The model under review builds one solid part; all positions refer to its coordinate system, in mm. Coordinates: 2 decimals unless noted, no trailing zeros. Write each loop counter-clockwise with the first axis right and the second up, starting at its lowest first coordinate (ties: lowest second). Pieces come first, ordered by that corner, then holes. Notation, with made-up numbers: (-2, -17.75) - (43, -17.75) arc R7 cw to (43, -11.75) - close; hole circle Ø5 at (16, -24.5). An arc over 180 degrees is marked (long way). Put each result on its own line as item: value.
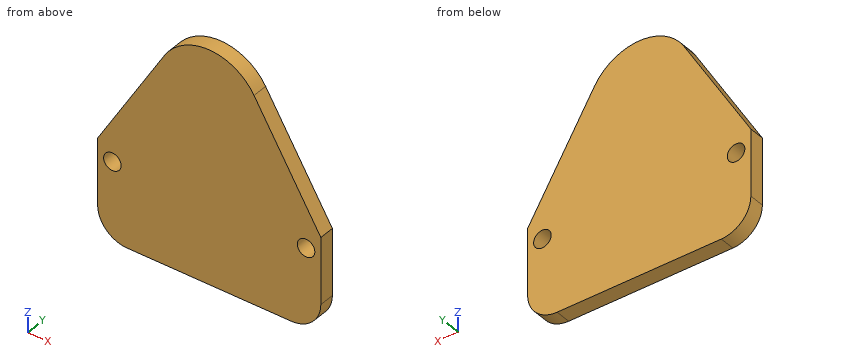
from build123d import *

# Parameters (mm, degrees)
SKETCH1_R           = 2.375
BOSS_EXTRUDE1_DEPTH = 4.15


with BuildPart() as part:
    # Sketch1 → Boss-Extrude1 (new body)
    with BuildSketch(Plane(origin=(0, 0, 0), x_dir=(1, 0, 0), z_dir=(0, 1, 0))):
        with BuildLine():
            Line((-22.25, 31.5), (22.25, 31.5))
            ThreePointArc((22.25, 31.5), (27.906854249, 29.156854249), (30.25, 23.5))
            Line((30.25, 23.5), (30.25, 5.5))
            Line((30.25, 5.5), (12.147813291, -24.627097925))
            ThreePointArc((12.147813291, -24.627097925), (0, -31.5), (-12.147813291, -24.627097925))
            Line((-12.147813291, -24.627097925), (-30.25, 5.5))
            Line((-30.25, 5.5), (-30.25, 23.5))
            ThreePointArc((-30.25, 23.5), (-27.906854249, 29.156854249), (-22.25, 31.5))
        make_face()
        with Locations(Location((26.25, 10.1, 0), (0, 0, 90))):
            Circle(SKETCH1_R, mode=Mode.SUBTRACT)
        with Locations(Location((-26.25, 10.1, 0), (0, 0, 90))):
            Circle(SKETCH1_R, mode=Mode.SUBTRACT)
    extrude(amount=BOSS_EXTRUDE1_DEPTH)


solid = part.part
1. Consider section C-C on x = 26.25. State the section outline as (y, z) points (3 decimals), plus the area to 3 significant figures.
Determined:
outline: (0, -30.428) - (4.15, -30.428) - (4.15, -12.475) - (0, -12.475) - close; (0, -7.725) - (4.15, -7.725) - (4.15, 1.157) - (0, 1.157) - close
area: 111 mm^2
2. For pin 1 Ø2 at (y, z) = (3, 24.5) entering from +X; pin 2 Ø4.5 at (x, z) = (26.25, -10.1) entering from +Y, all flat-tipped, find the tip position at first contact; note any pin that passes through.
Determined:
pin 1: stops at x = 12.83
pin 2: passes through
3. To check wall thickness, follow probe 1 along X at (y, z) = (1.15, -10.1) (3 decimals); probe 2 along Z at (x, y) = (24.5, 1.2); probe 3 along Z at (x, y) = (-26.25, 1.3) (3 decimals). State the ranges of each line that lie inside material, in increasing order.
Determined:
probe 1: x = -30.25 to -28.625, -23.875 to 23.875, 28.625 to 30.25
probe 2: z = -31.18 to -11.71, -8.49 to 4.07
probe 3: z = -30.428 to -12.475, -7.725 to 1.157
4. Consider section D-D on x = -25. State the section outline as (y, z) points, plus the area to 3 significant figures.
Determined:
outline: (0, -31.01) - (4.15, -31.01) - (4.15, -12.12) - (0, -12.12) - close; (0, -8.08) - (4.15, -8.08) - (4.15, 3.24) - (0, 3.24) - close
area: 125 mm^2
5. Consider section A-A on y = 1.85. State the section outline as (x, z) points (3 decimals).
Determined:
outline: (-30.25, -23.5) arc R8 ccw to (-22.25, -31.5) - (22.25, -31.5) arc R8 ccw to (30.25, -23.5) - (30.25, -5.5) - (12.148, 24.627) arc R14.172 ccw to (-12.148, 24.627) - (-30.25, -5.5) - close; hole circle Ø4.75 at (-26.25, -10.1); hole circle Ø4.75 at (26.25, -10.1)
6. Consider section B-B on z = -10.1. State the section outline as (x, y) points (3 decimals), plus the area to 3 significant figures.
Determined:
outline: (-30.25, 0) - (-28.625, 0) - (-28.625, 4.15) - (-30.25, 4.15) - close; (-23.875, 0) - (23.875, 0) - (23.875, 4.15) - (-23.875, 4.15) - close; (28.625, 0) - (30.25, 0) - (30.25, 4.15) - (28.625, 4.15) - close
area: 212 mm^2
